Check sheet for the modelled part. Datum: model origin and axes. Units: mm. Round coordinates to 2 decimals unless told otherwise and drop trailing zeros. Order: outer loops, then holes, each group sorted by start corner. A loop starts at its lowest first (then second) coordinate and runs counter-clockwise, first axis right, second up.
Q1. Scan lines: probe 1 along Z at (x, y) = (0.7, 8); probe 2 along Z at (x, y) = (0.9, 7.25); probe 3 along Y at (x, z) = (1.1, -4.25). Record each from-to range of solid material in increasing order.
Q2. Cross-section at D-D on z = 0.5. Record the cut outline in (x, y).
Q3. Cross-section at A-A on z = -4.25. Record the cut outline in (x, y), then the cut area to 3 significant figures.
Q4. Cross-section at B-B on x = 0.25. Record the cut outline in (y, z), then the cut area to 3 significant figures.
Q5. Cross-section at C-C on y = 6.5. Record the cut outline in (x, z).
Autodesk Inventor part; units mm, degrees
ref_plane "YZ Plane" through (0, 0, 0) normal (1, 0, 0) x (0, 1, 0)
ref_plane "XZ Plane" through (0, 0, 0) normal (0, 1, 0) x (-1, 0, 0)
ref_plane "XY Plane" through (0, 0, 0) normal (0, 0, 1) x (1, 0, 0)
sketch "スケッチ1" plane through (0, 0, 0) normal (1, 0, 0) x (0, 1, 0)
  line L0 (12, 0) -> (0, 0)
  line L1 (0, 0) -> (0, -25)
  line L2 (0, -25) -> (12, -25)
  line L3 (12, -25) -> (12, 0)
  line L4 (12, 0) -> (0, 5.5957)
  line L5 (0, 5.5957) -> (0, 0)
  line L6 (12, -20) -> (0, -16.7846)
  line L7 (8, -18.9282) -> (12, -16.6188)
  dimension "d11" = 12
  dimension "d12" = 25
  dimension "d14" = 25
  dimension "d15" = 15
  dimension "d16" = 5
  dimension "d17" = 45
  dimension "d18" = 4
extrude "プレート1" add sketch "スケッチ1" along normal blind 1.5 contours L3 L7 L6 L1 L0 | L0 L5 L4
sketch "スケッチ3" plane through (0, 0, 0) normal (-1, 0, 0) x (0, 0, 1)
  circle A0 centre (-6.7433, 7.5315) radius 0.8
  circle A1 centre (-14.5922, 3.8716) radius 0.8
  circle A2 centre (-9.6112, 3.4358) radius 0.8
  circle A3 centre (-4.6303, 3) radius 0.8
  line L0 (-14.5922, 3.8716) -> (-9.6112, 3.4358) construction
  line L1 (-9.6112, 3.4358) -> (-4.6303, 3) construction
  line L2 (-6.7433, 7.5315) -> (-4.6303, 3) construction
  line L3 (0, 12) -> (5.5957, 0)
  line L4 (-6.7433, 7.5315) -> (-7.1207, 3.2179) construction
  line L5 (-11.7243, 7.9673) -> (-12.1017, 3.6537) construction
  line L6 (-11.7243, 7.9673) -> (-6.7433, 7.5315) construction
  circle A4 centre (-11.7243, 7.9673) radius 0.8
  line L7 (-6.7433, 7.5315) -> (-4.8683, 8.4059) construction
  line L8 (5.5957, 0) -> (-16.7846, 0)
  point P0 (0, 0)
  dimension "d23" = 1.6
  dimension "d26" = 5
  dimension "d29" = 5
  dimension "d30" = 8
  dimension "d31" = 3
extrude "切り取り1" cut sketch "スケッチ3" against normal blind 1.5
chamfer "面取り1" distance 3 angle 45 1 edges at (0.75, 12, 0)
equation "\"d29\" = d26"
equation "\"d32\" = Thickness"
equation "\"d0\" = Thickness"
equation "\"BendRadius\" = Thickness"
equation "\"BendReliefWidth\" = Thickness"
equation "\"BendReliefDepth\" = 0.5 * Thickness"
equation "\"CornerReliefSize\" = 4 * Thickness"
equation "\"MinimumRemnant\" = 2 * Thickness"
equation "\"TransitionRadius\" = BendRadius"
equation "\"JacobiRadiusSize\" = BendRadius"
equation "\"GapSize\" = Thickness"
properties part number "face_gard_right" material "アルミニウム 6061"
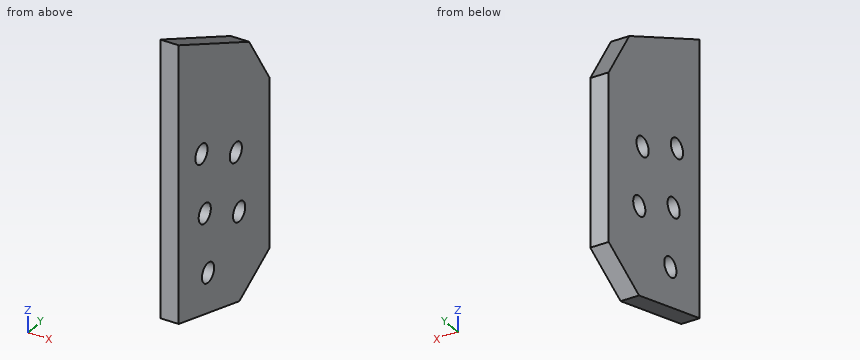
Results found:
1. probe 1: z = -18.93 to -12.52, -10.92 to -7.39, -6.09 to 1.87
1. probe 2: z = -18.73 to -12.08, -11.37 to -7.49, -5.99 to 2.21
1. probe 3: y = 0 to 2.3, 3.7 to 12
2. outline: (0, 0) - (1.5, 0) - (1.5, 9.77) - (0, 9.77) - close
3. outline: (0, 0) - (1.5, 0) - (1.5, 2.3) - (0, 2.3) - close; (0, 3.7) - (1.5, 3.7) - (1.5, 12) - (0, 12) - close
3. area: 15.9 mm2
4. outline: (0, -16.78) - (8, -18.93) - (12, -16.62) - (12, -3) - (9.28, 1.27) - (0, 5.6) - close; hole circle Ø1.6 at (3, -4.63); hole circle Ø1.6 at (3.44, -9.61); hole circle Ø1.6 at (3.87, -14.59); hole circle Ø1.6 at (7.53, -6.74); hole circle Ø1.6 at (7.97, -11.72)
4. area: 233 mm2
5. outline: (0, -18.53) - (1.5, -18.53) - (1.5, 2.56) - (0, 2.56) - close
